Build history of the part. All positions in model axes, mm. A direction names the side the tool comes from. Give positions to 0.01 mm unless a question says otherwise; leave off trailing zeros. Write each loop counter-clockwise with the first axis right and the second up, starting at its lowest first coordinate (ties: lowest second). Pieces come first, ordered by that corner, then holes. Notation, with made-up numbers: (87, -30) -> (95, -30) arc R13 ccw to (95, -10) -> close; hole circle Ø10 at (73, -34.75). An arc over 180 degrees is marked (long way). Put each result on its own line as item: value. Start each with the question number.
Item 1: Two-plate mould, pull along Z, no slides. Class faces 1 (the cylindrical face through (12.6, 1.52, 13.64)), 2 (the cylindrical face through (-11.98, 32.1, -13.64)), 3 (the cylindrical face through (-12.02, 26.92, -9.58)), 4 (the cylindrical face through (-12.02, 14.36, -0.26)): pulls with the +Z half, pulls with the -Z half, needs draft (parallel to the pull), parting line crosses it, or undercut.
Item 2: Flat gauge pins, fed straight in: pin 1 Ø5 at (y, z) = (20, -8.5) entering from +X; pin 2 Ø3 at (y, z) = (12.375, -9.15) entering from -X; pin 3 Ø8 at (x, z) = (-4.5, -4) entering from -Y; pin 4 Ø10 at (x, z) = (9.5, 0) entering from +Y. Where does each tip first touch, or does it go through?
Item 3: Drill centre lines: line 1 along Z through (x, y) = (8.25, 1.65); line 2 along Z through (x, y) = (0, 1.15) (3 decimals); line 3 along Y through (x, z) = (12.5, -3.75). Where is each one in solid material? Low to high.
Item 4: Slice it at A-A, the plane x = 3. List the corners of the cut face in (y, z) (3 decimals).
Item 5: Slice it at C-C, the plane x = 8.25. List the corners of the cut face in (y, z), plus the area to 3 significant figures.
Item 6: Slice it at B-B, the plane z = 9.15. List the corners of the cut face in (x, y) (3 decimals), plus the area to 3 significant figures.
Item 7: Tool access for faces 5 (the flat face through (-8, 8, 12.5)), 6 (the flat face through (-12, 15, 0)), 7 (the flat face through (0, 1, 5.625)): list every direction of +Z, -Z, +X, -X, +Y, -Y with a clear straight run to the whole face (end or side of a thin tool).
Item 8: Slice it at D-D, the plane z = -5. List the corners of the cut face in (x, y) (3 decimals), plus the area to 4 significant figures.
Autodesk Inventor part; units mm, degrees
ref_plane "YZ Plane" through (0, 0, 0) normal (1, 0, 0) x (0, 1, 0)
ref_plane "XZ Plane" through (0, 0, 0) normal (0, 1, 0) x (-1, 0, 0)
ref_plane "XY Plane" through (0, 0, 0) normal (0, 0, 1) x (1, 0, 0)
sketch "Sketch1" plane through (0, 0, 0) normal (0, 1, 0) x (-1, 0, 0)
  line L0 (13.5, 14.5) -> (-13.5, 14.5)
  line L1 (-13.5, 14.5) -> (-13.5, -14.5)
  line L2 (-13.5, -14.5) -> (13.5, -14.5)
  line L3 (13.5, -14.5) -> (13.5, 14.5)
  line L4 (5.625, 5.625) -> (-5.625, 5.625)
  line L5 (-5.625, 5.625) -> (-5.625, -5.625)
  line L6 (-5.625, -5.625) -> (5.625, -5.625)
  line L7 (5.625, -5.625) -> (5.625, 5.625)
  circle A0 centre (-8.25, 0) radius 2
  circle A1 centre (-8.25, -9.15) radius 2
  line L8 (-8.25, 0) -> (-4.1919, 0) construction
  circle A2 centre (-8.25, 9.15) radius 2
  line L9 (-4.125, 12.0498) -> (-4.125, -8.6633) construction
  circle A3 centre (0, -9.15) radius 2
  circle A4 centre (0, 9.15) radius 2
  point P0 (0, 0)
  point P1 (-4.125, 1.6932)
  dimension "d0" = 29
  dimension "d1" = 27
  dimension "d2" = 13.5
  dimension "d3" = 14.5
  dimension "d4" = 11.25
  dimension "d5" = 11.25
  dimension "d6" = 5.625
  dimension "d7" = 5.625
  dimension "d8" = 4
  dimension "d9" = 5.25
  dimension "d10" = 4
  dimension "d12" = 5.35
  dimension "d13" = 4.125
  dimension "d23" = 2.625
  dimension "d40" = 9.15
  dimension "d41" = 8.25
extrude "Extrusion1" add sketch "Sketch1" along normal blind 3
fillet "Fillet1" radius 3 2 edges at (13.5, 1.5, 14.5) (13.5, 1.5, -14.5)
sketch "Sketch2" plane through (-13.5, 0, -14.5) normal (-1, 0, 0) x (0, 0, 1)
  line L0 (0, 0) -> (0, 3)
  line L1 (0, 0) -> (29, 0)
  line L2 (29, 0) -> (29, 33)
  line L3 (29, 33) -> (0, 33)
  line L4 (0, 33) -> (0, 0)
  line L5 (0, 3) -> (29, 3)
  line L6 (8.875, 26.25) -> (20.125, 26.25)
  line L7 (20.125, 26.25) -> (20.125, 15)
  line L8 (20.125, 15) -> (8.875, 15)
  line L9 (8.875, 15) -> (8.875, 26.25)
  circle A0 centre (14.5, 12.375) radius 2
  circle A1 centre (23.65, 12.375) radius 2
  line L10 (3.2403, 20.625) -> (27.5408, 20.625) construction
  line L11 (14.5, 12.375) -> (14.5, 30.5106) construction
  circle A2 centre (5.35, 12.375) radius 2
  circle A3 centre (14.5, 28.875) radius 2
  circle A4 centre (23.65, 28.875) radius 2
  circle A5 centre (5.35, 28.875) radius 2
  line L12 (2.8915, 16.5) -> (25.3317, 16.5) construction
  circle A6 centre (23.65, 28.875) radius 2
  circle A7 centre (5.35, 28.875) radius 2
  circle A8 centre (23.65, 20.625) radius 2
  circle A9 centre (5.35, 20.625) radius 2
  point P0 (14.5, 0)
  dimension "d17" = 29
  dimension "d18" = 33
  dimension "d19" = 11.25
  dimension "d20" = 11.25
  dimension "d21" = 12
  dimension "d22" = 8.875
  dimension "d24" = 4
  dimension "d25" = 2.625
  dimension "d26" = 4
  dimension "d27" = 5.35
  dimension "d28" = 0
  dimension "d29" = 5.625
  dimension "d30" = 5.625
  dimension "d31" = 8.25
  dimension "d32" = 4.125
extrude "Extrusion2" add sketch "Sketch2" against normal blind 3 contours L4 L3 L2 L5
fillet "Fillet2" radius 3 2 edges at (-12, 33, 14.5) (-12, 33, -14.5)
sketch "Sketch3" plane through (-13.5, 0, 14.5) normal (0, 0, 1) x (1, 0, 0)
  line L0 (0, 18.625) -> (0, 22.625)
  line L1 (11.5, 3) -> (15.5, 3)
  line L2 (3, 22.625) -> (3, 18.625)
  line L3 (3, 22.625) -> (3, 18.625)
  line L4 (3, 20.625) -> (13.5, 3)
  line L5 (19.125, 3) -> (7.875, 3)
  line L6 (3, 30) -> (3, 3)
  line L7 (3, 3) -> (24, 3)
  point P0 (13.5, 0)
extrude "Extrusion3" add sketch "Sketch3" against normal blind 2
sketch "Sketch4" plane through (10.5, 0, -14.5) normal (0, 0, -1) x (-1, 0, 0)
  line L0 (10.5, 3) -> (21, 20.625)
  line L1 (21, 20.625) -> (21, 3)
  line L2 (21, 3) -> (10.5, 3)
  point P0 (10.5, 0)
extrude "Extrusion4" add sketch "Sketch4" against normal blind 2
equation "\"d5\" = d4"
equation "\"d20\" = d19"
equation "\"d22\" = 0.5 * d17 - 0.5 * d19"
equation "\"d26\" = d24"
equation "\"d29\" = 0.5 * d20"
equation "\"d30\" = d29"
equation "\"d32\" = 0.5 * d31"
properties part number "SoporteUnion" material "Plastic, Opaque Black"
Values follow:
1. face 1: pulls with the +Z half
1. face 2: pulls with the -Z half
1. face 3: undercut
1. face 4: undercut
2. pin 1: x = -10.5
2. pin 2: through
2. pin 3: y = 0
2. pin 4: y = 3
3. line 1: -14.5 to -11.15, -7.15 to -2, 2 to 7.15, 11.15 to 14.5
3. line 2: -14.5 to -11.15, -7.15 to -5.625, 5.625 to 7.15, 11.15 to 14.5
3. line 3: 0 to 3
4. outline: (0, -14.5) -> (3, -14.5) -> (3, -5.625) -> (0, -5.625) -> close; (0, 5.625) -> (3, 5.625) -> (3, 14.5) -> (0, 14.5) -> close
5. outline: (0, -14.5) -> (3, -14.5) -> (3, -11.15) -> (0, -11.15) -> close; (0, -7.15) -> (3, -7.15) -> (3, -2) -> (0, -2) -> close; (0, 2) -> (3, 2) -> (3, 7.15) -> (0, 7.15) -> close; (0, 11.15) -> (3, 11.15) -> (3, 14.5) -> (0, 14.5) -> close
5. area: 51.0 mm2
6. outline: (-13.5, 0) -> (-2, 0) -> (-2, 3) -> (-10.5, 3) -> (-10.5, 10.375) -> (-13.5, 10.375) -> close; (-13.5, 14.375) -> (-10.5, 14.375) -> (-10.5, 18.625) -> (-13.5, 18.625) -> close; (-13.5, 22.625) -> (-10.5, 22.625) -> (-10.5, 26.875) -> (-13.5, 26.875) -> close; (-13.5, 30.875) -> (-10.5, 30.875) -> (-10.5, 33) -> (-13.5, 33) -> close; (2, 0) -> (6.25, 0) -> (6.25, 3) -> (2, 3) -> close; (10.25, 0) -> (13.5, 0) -> (13.5, 3) -> (10.25, 3) -> close
6. area: 111 mm2
7. face 5: +X, +Y
7. face 6: +X, -X
7. face 7: +Y, -Y
8. outline: (-13.5, 0) -> (-5.625, 0) -> (-5.625, 3) -> (-10.5, 3) -> (-10.5, 15) -> (-13.5, 15) -> close; (-13.5, 26.25) -> (-10.5, 26.25) -> (-10.5, 33) -> (-13.5, 33) -> close; (5.625, 0) -> (13.5, 0) -> (13.5, 3) -> (5.625, 3) -> close
8. area: 103.5 mm2
